from build123d import *

# Parameters (mm, degrees)
SKETCH1_W           = 12.7
SKETCH1_H           = 30
SKETCH1_W_2         = 55.36
SKETCH1_H_2         = 12.7
BOSS_EXTRUDE1_DEPTH = 12.7
SKETCH3_W           = 25
SKETCH3_H           = 12.7
CUT_EXTRUDE2_DEPTH  = 300.216536308
SKETCH2_R           = 3.2
CUT_EXTRUDE1_DEPTH  = 300.216536308


with BuildPart() as part:
    # Sketch1 → Boss-Extrude1 (new body)
    with BuildSketch(Plane.XY):
        Polygon((221.23, 144.4), (221.23, 131.7), (254.34, 131.7), (254.34, 78.5), (221.23, 78.5), (221.23, 65.8), (254.34, 65.8), (254.34, 12.7), (221.23, 12.7), (221.23, 0), (181.23, 0), (181.23, 12.7), (125.87, 12.7), (125.87, 0), (-5, 0), (-5, 144.4), (0, 144.4), (25.29, 144.4), (25.29, 157.1), (50.29, 157.1), (50.29, 144.4), (75.58, 144.4), (75.58, 157.1), (100.58, 157.1), (100.58, 144.4), (125.87, 144.4), (125.87, 131.7), (181.23, 131.7), (181.23, 144.4), align=None)
        with Locations((6.35, 111.7)):
            Rectangle(SKETCH1_W, SKETCH1_H, mode=Mode.SUBTRACT)
        with Locations((6.35, 20)):
            Rectangle(SKETCH1_W, SKETCH1_H, mode=Mode.SUBTRACT)
        with Locations((153.55, 72.15)):
            Rectangle(SKETCH1_W_2, SKETCH1_H_2, mode=Mode.SUBTRACT)
    extrude(amount=BOSS_EXTRUDE1_DEPTH)

    # Sketch3 → Cut-Extrude2 (cut, through all)
    with BuildSketch(Plane.XY.offset(12.7)):
        with Locations((37.79, 6.35)):
            Rectangle(SKETCH3_W, SKETCH3_H)
        with Locations((88.08, 6.35)):
            Rectangle(SKETCH3_W, SKETCH3_H)
    extrude(amount=-CUT_EXTRUDE2_DEPTH, mode=Mode.SUBTRACT)

    # Sketch2 → Cut-Extrude1 (cut, through all)
    with BuildSketch(Plane.XY.offset(12.7)):
        with Locations((129.07, 131.7)):
            Circle(SKETCH2_R)
        with Locations((178.03, 131.7)):
            Circle(SKETCH2_R)
        with Locations((224.43, 131.7)):
            Circle(SKETCH2_R)
        with Locations((224.43, 78.5)):
            Circle(SKETCH2_R)
        with Locations((224.43, 65.8)):
            Circle(SKETCH2_R)
        with Locations((224.43, 12.7)):
            Circle(SKETCH2_R)
        with Locations((28.49, 12.7)):
            Circle(SKETCH2_R)
        with Locations((47.09, 12.7)):
            Circle(SKETCH2_R)
        with Locations((178.03, 12.7)):
            Circle(SKETCH2_R)
        with Locations((178.03, 65.8)):
            Circle(SKETCH2_R)
        with Locations((178.03, 78.5)):
            Circle(SKETCH2_R)
        with Locations((129.07, 78.5)):
            Circle(SKETCH2_R)
        with Locations((129.07, 65.8)):
            Circle(SKETCH2_R)
        with Locations((129.07, 12.7)):
            Circle(SKETCH2_R)
        with Locations((78.78, 12.7)):
            Circle(SKETCH2_R)
        with Locations((3.2, 126.7)):
            Circle(SKETCH2_R)
        with Locations((3.2, 96.7)):
            Circle(SKETCH2_R)
        with Locations((3.2, 35)):
            Circle(SKETCH2_R)
        with Locations((3.2, 5)):
            Circle(SKETCH2_R)
        with Locations((12.7, 8.2)):
            Circle(SKETCH2_R)
        with Locations((12.7, 31.8)):
            Circle(SKETCH2_R)
        with Locations((12.7, 99.9)):
            Circle(SKETCH2_R)
        with Locations((12.7, 123.5)):
            Circle(SKETCH2_R)
        with Locations((22.09, 144.4)):
            Circle(SKETCH2_R)
        with Locations((53.49, 144.4)):
            Circle(SKETCH2_R)
        with Locations((72.38, 144.4)):
            Circle(SKETCH2_R)
        with Locations((103.78, 144.4)):
            Circle(SKETCH2_R)
        with Locations((97.38, 12.7)):
            Circle(SKETCH2_R)
    extrude(amount=-CUT_EXTRUDE1_DEPTH, mode=Mode.SUBTRACT)


solid = part.part
Design review of the part built by this model. Coordinates are the model's own, in mm. A direction names the side the tool comes from. Round coordinates to 2 decimals unless told otherwise and drop trailing zeros. Write each loop counter-clockwise with the first axis right and the second up, starting at its lowest first coordinate (ties: lowest second). Pieces come first, ordered by that corner, then holes. Notation, with made-up numbers: (69, -38.75) - (85, -38.75) arc R11 cw to (85, -33.75) - close; hole circle Ø3 at (22, -19). An arc over 180 degrees is marked (long way). Use a Markdown table: item, result. Add a question column.
1. For faces 1 (the face through (88, 12.7, 6)), 2 (the face through (25.29, 151, 6)), 3 (the face through (241, 12.7, 6)), 4 (the face through (221.23, 72, 6)), 5 (the face through (12.7, 20, 6)), list the 3-axis set-ups (+Z, -Z, +X, -X, +Y, -Y) from which the entire face can be reached by the end or side of a thin tool; tool diameter is ignored.
2. Mouldability with a two-part tool opening along Y and no side actions: class faces 6 (the face through (125.87, 6, 6)), 7 (the face through (72.3, 141.2, 6.4)), 8 (the face through (224.5, 81.7, 6.4)), 9 (the face through (47.2, 15.9, 6.4)) as +Y half, -Y half, draft (parallel to the pull), parting line (faces both ways), or undercut.
3. We need section D-D (x = 22.09). State the section outline as (y, z) points, then the cut area to 3 significant figures.
4. We need section C-C (z = 2). Count the separate pieces of the cut face and the enclosed holes in it, then the cut area to 3 significant figures.
5. We need section A-A (y = 148). State the section outline as (x, z) points, then the cut area to 3 significant figures.
6. We need section B-B (x = 178.03). State the section outline as (y, z) points, then the cut area to 3 significant figures.
7. Clearance check with flat-ended pins moving along their axes: pin 1 (4 mm diameter, centred on y = 138.5, z = 9, fed in from +X); pin 2 (6 mm diameter, centred on x = 155, z = 7, fed in from -Y); pin 3 (1 mm diameter, centred on x = 186.5, y = 122, fed in from -Z); pin 4 (6 mm diameter, centred on x = 62.5, z = 4.5, fed in from +Y). State where each tip first meets the part, or that it passes through.
8. Wall thickness on probe 1 along Y at (x, z) = (164, 6.75); probe 2 along X at (y, z) = (132.5, 1.5); probe 3 along X at (y, z) = (131, 10): over which ranges is each line inside the solid? List them lowest first.
Output:
| question | item | result |
|---|---|---|
| 1 | face 1 | +Z, -Z, -Y |
| 1 | face 2 | +Z, -Z, -X, +Y |
| 1 | face 3 | +Z, -Z, +X, -Y |
| 1 | face 4 | +Z, -Z, +X |
| 1 | face 5 | +Z, -Z |
| 2 | face 6 | draft |
| 2 | face 7 | +Y half |
| 2 | face 8 | undercut |
| 2 | face 9 | -Y half |
| 3 | outline | (0, 0) - (141.2, 0) - (141.2, 12.7) - (0, 12.7) - close |
| 3 | area | 1,790 mm2 |
| 4 | separate pieces | 1 |
| 4 | enclosed holes | 3 |
| 4 | area | 32,900 mm2 |
| 5 | outline | (25.29, 0) - (50.29, 0) - (50.29, 12.7) - (25.29, 12.7) - close; (75.58, 0) - (100.58, 0) - (100.58, 12.7) - (75.58, 12.7) - close |
| 5 | area | 635 mm2 |
| 6 | outline | (15.9, 0) - (62.6, 0) - (62.6, 12.7) - (15.9, 12.7) - close; (81.7, 0) - (128.5, 0) - (128.5, 12.7) - (81.7, 12.7) - close |
| 6 | area | 1,190 mm2 |
| 7 | pin 1 | stops at x = 221.23 |
| 7 | pin 2 | stops at y = 12.7 |
| 7 | pin 3 | stops at z = 0 |
| 7 | pin 4 | stops at y = 144.4 |
| 8 | probe 1 | y = 12.7 to 65.8, 78.5 to 131.7 |
| 8 | probe 2 | x = -5 to 125.87, 181.23 to 221.23 |
| 8 | probe 3 | x = -5 to 125.95, 132.19 to 174.91, 181.15 to 221.31, 227.55 to 254.34 |
